Geometry: see drawing. Coordinates: mm, zero at the bounding-box minimum. Coordinates: 2 decimals unless noted, no trailing zeros. Write each loop counter-clockwise with the first axis right and the second up, starting at its lowest first coordinate (ties: lowest second). Pieces come first, ordered by that corner, then holes. Notation, with made-up numbers: M 88.5,34.5 L 114.5,34.5 A17 cw 114.5,43.5 Z; hole C 45.25,7 d10. An arc over 180 degrees is marked long. One line per item, written item: value. Start each with the question number.
Item 1: Pin query (flat end, axial travel): P1, Ø1, axis at x = 97.5, z = 5, coming from the -Y side; P2, Ø3, axis at y = 3, z = 2, coming from the +X side; P3, Ø1.3, axis at x = 212.5, y = 5, coming from the -Z side. Return the tip coordinate at first contact, or that it passes through.
Item 2: Ray query, L1, parallel to X at y = 1.25, z = 5.25; L2, parallel to X at y = 5.5, z = 4.5 (1 decimal); L3, parallel to Y at x = 163, z = 5. Return the intervals inside material, ascending. Write a range as from..to.
Item 3: Cut plane B-B, the plane x = 110.5. Output: boundary loops of the cut face in (y, z), then the cut area to 3 significant figures.
Item 4: Cut plane A-A, the plane z = 1.5. Output: boundary loops of the cut face in (x, y).
Item 5: Cut plane D-D, the plane x = 21.5. Output: boundary loops of the cut face in (y, z).
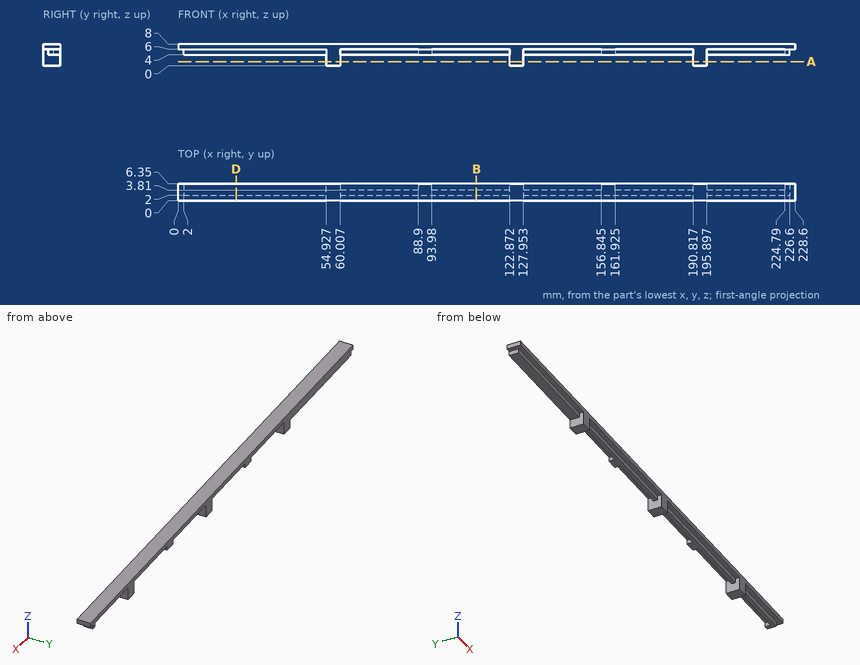
From the geometry:
1. P1: stops at y = 2
1. P2: stops at x = 195.9
1. P3: stops at z = 6
2. L1: x = 54.93..60.01, 122.87..127.95, 190.82..195.9
2. L2: x = 2..60, 88.9..94, 122.9..128, 156.8..161.9, 190.8..195.9, 224.8..226.6
2. L3: y = 2..3.81
3. outline: M 0,6 L 2,6 L 2,4 L 3.81,4 L 3.81,6 L 6.35,6 L 6.35,8 L 0,8 Z
3. area: 16.3 mm²
4. outline: M 54.93,0 L 60.01,0 L 60.01,6.35 L 54.93,6.35 Z; M 122.87,0 L 127.95,0 L 127.95,6.35 L 122.87,6.35 Z; M 190.82,0 L 195.9,0 L 195.9,6.35 L 190.82,6.35 Z
5. outline: M 0,6 L 2,6 L 2,4 L 6.35,4 L 6.35,8 L 0,8 Z
